Can you work these out from the model? Positions are in its coordinate system, mm. Face numbers are marked on the shaded views. A direction names the side the tool comes from. Give positions to 0.01 mm unless a question says otherwise; leave off trailing zeros. Loops run counter-clockwise (first coordinate to the right, second up) from the corner with the lowest first, then second, coordinate; pieces in that order, holes last. Notation, with made-up numbers: (75.5, 47.25) - (94.5, 47.25) arc R32 cw to (94.5, 86.25) - close; hole circle Ø10 at (11.25, -7). An arc over 180 degrees is marked (long way). Write item = value, one per line.
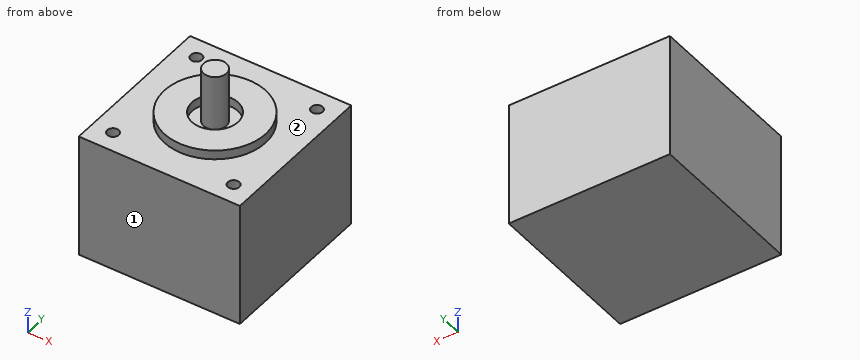
from build123d import *

# Parameters (mm, degrees)
F0_W     = 35
F0_H     = 35
F1_DEPTH = 27
F2_R     = 11
F2_R_2   = 5
F3_DEPTH = 2
F4_R     = 2.5
F5_DEPTH = 12
F7_D     = 2.5
F7_DEPTH = 13.5
F7_TIP   = 0.7510757738


with BuildPart() as f1:
    # F0 (on Top) → F1 (new body)
    with BuildSketch(Plane.XY):
        Rectangle(F0_W, F0_H)
    extrude(amount=F1_DEPTH)

    # F2 (on face) → F3 (join)
    with BuildSketch(Plane.XY.offset(27)):
        Circle(F2_R)
        Circle(F2_R_2, mode=Mode.SUBTRACT)
    extrude(amount=F3_DEPTH)

    # F4 (on face) → F5 (join)
    with BuildSketch(Plane.XY.offset(27)):
        Circle(F4_R)
    extrude(amount=F5_DEPTH)

    # F7
    with Locations(Plane.XY.offset(27)):
        with Locations((-13.1, 13.1), (13.1, 13.1), (13.1, -13.1), (-13.1, -13.1)):
            Hole(F7_D / 2, depth=F7_DEPTH)
            with Locations((0, 0, -(F7_DEPTH + F7_TIP / 2))):  # 118° drill point
                Cone(0, F7_D / 2, F7_TIP, mode=Mode.SUBTRACT)


solid = f1.part
Q1. Imagine slicing it at C-C, the plane x = -6. Write out the boundary of the cut face in (y, z), then the cut area to 3 significant figures.
Output:
outline = (-17.5, 0) - (17.5, 0) - (17.5, 27) - (9.22, 27) - (9.22, 29) - (-9.22, 29) - (-9.22, 27) - (-17.5, 27) - close
area = 982 mm2
Q2. For pin 1 (5 mm diameter, centred on x = -5.5, y = 13, fed in from +Z); pin 2 (2 mm diameter, centred on x = -13.1, y = -13.1, fed in from +Z); pin 3 (1.5 mm diameter, centred on x = 5.5, z = 28, fed in from -Y); pin 4 (1 mm diameter, centred on x = 9.5, z = 30, fed in from +Y), each with a flat end and sliding along its axis, tell me the tip position at first contact or that it passes through.
Output:
pin_1 = 27
pin_2 = 13.35
pin_3 = -9.92
pin_4 = through
Q3. I need wall thicknesses on L1, parallel to X at y = -13, z = 22; L2, parallel to Z at x = 10, y = -11.5. Which ranges of each line are inside material? Lowest first, please.
Output:
L1 = -17.5 to -14.35, -11.85 to 11.85, 14.35 to 17.5
L2 = 0 to 27
Q4. Imagine slicing it at A-A, the plane z = 28. Write out the boundary of the cut face in (x, y), then the cut area to 3 significant figures.
Output:
outline = circle Ø22 at (0, 0); circle Ø5 at (0, 0); hole circle Ø10 at (0, 0)
area = 321 mm2
Q5. Which directions (+Z, -Z, +X, -X, +Y, -Y) give clear straight access to the entire face, cutting with the end or side of a thin tool? Please do the marked faces 1 and 2.
Output:
face_1 = +Z, -Z, +X, -X, -Y
face_2 = +Z
Q6. Imagine slicing it at B-B, the plane y = 0. Write out the boundary of the cut face in (x, z), then the cut area to 3 significant figures.
Output:
outline = (-17.5, 0) - (17.5, 0) - (17.5, 27) - (11, 27) - (11, 29) - (5, 29) - (5, 27) - (2.5, 27) - (2.5, 39) - (-2.5, 39) - (-2.5, 27) - (-5, 27) - (-5, 29) - (-11, 29) - (-11, 27) - (-17.5, 27) - close
area = 1,030 mm2
